The figure shows three views and two pictorial views of one solid part (mm, origin at its lowest corner). Answer the questions. Coordinates: 2 decimals unless noted, no trailing zeros. Write each loop counter-clockwise with the first axis right and the second up, starting at its lowest first coordinate (ties: lowest second). Pieces come first, ordered by that corner, then holes.
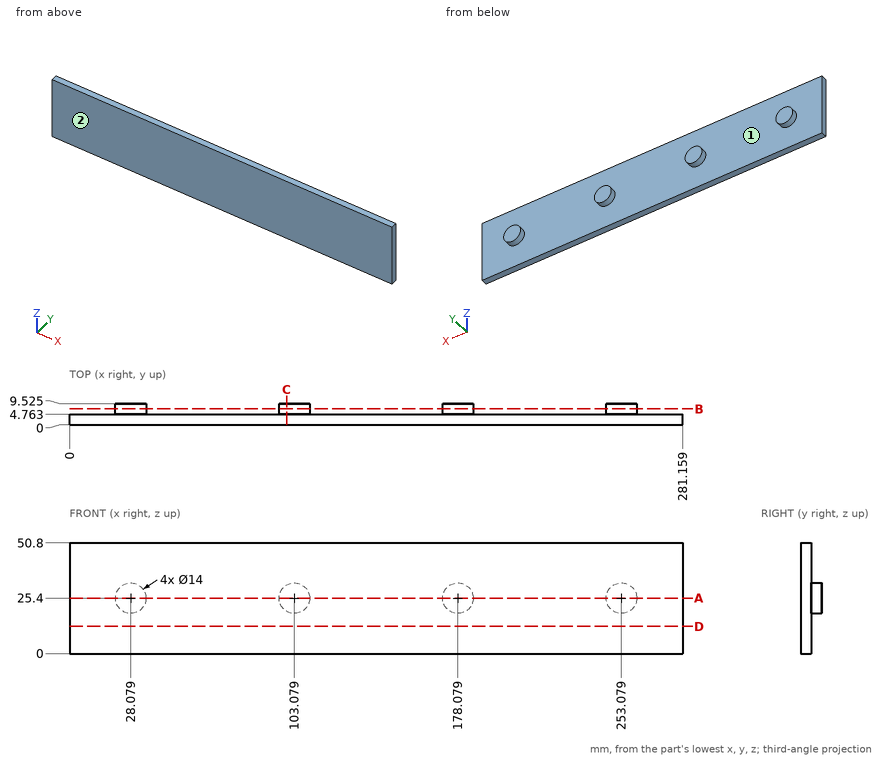
1. Find the intervals of material crossed by L1, parallel to Y at x = 124, z = 44; L2, parallel to Z at x = 257.5, y = 7.5 (1 decimal), in increasing order.
Results found:
L1: y = 0 to 4.76
L2: z = 20 to 30.8
2. Section A-A on z = 25.4 is taken. Give the vertices of the cut face in (x, y) (1 decimal), then the cut area to 3 significant figures.
Results found:
outline: (0, 0) - (281.2, 0) - (281.2, 4.8) - (260.1, 4.8) - (260.1, 9.5) - (246.1, 9.5) - (246.1, 4.8) - (185.1, 4.8) - (185.1, 9.5) - (171.1, 9.5) - (171.1, 4.8) - (110.1, 4.8) - (110.1, 9.5) - (96.1, 9.5) - (96.1, 4.8) - (35.1, 4.8) - (35.1, 9.5) - (21.1, 9.5) - (21.1, 4.8) - (0, 4.8) - close
area: 1,610 mm2
3. A flat-ended cylindrical pin translates along its axis: P1, Ø12, axis at x = 116.5, z = 31.5, coming from the +Y side. Find the tip coordinate at first contact, or state that the pin passes through.
Results found:
P1: stops at y = 4.76
4. Section B-B on y = 7.25 is taken. Give the vertices of the cut face in (x, z), then the cut area to 3 significant figures.
Results found:
outline: circle Ø14 at (28.08, 25.4); circle Ø14 at (103.08, 25.4); circle Ø14 at (178.08, 25.4); circle Ø14 at (253.08, 25.4)
area: 616 mm2
5. Section D-D on z = 12.5 is taken. Give the vertices of the cut face in (x, y), then the cut area to 3 significant figures.
Results found:
outline: (0, 0) - (281.16, 0) - (281.16, 4.76) - (0, 4.76) - close
area: 1,340 mm2
6. Section C-C on x = 99.5 is taken. Give the vertices of the cut face in (y, z) (1 decimal).
Results found:
outline: (0, 0) - (4.8, 0) - (4.8, 19.4) - (9.5, 19.4) - (9.5, 31.4) - (4.8, 31.4) - (4.8, 50.8) - (0, 50.8) - close
7. For a pull along X with two mould halves and no side action, classify the marked faces 1 and 2 as pulls with the +X half, pulls with the -X half, needs draft (parallel to the pull), parting line crosses it, or undercut.
Results found:
face 1: undercut
face 2: needs draft
